```python
from build123d import *

# Parameters (mm, degrees)
SKETCH1_W               = 45
SKETCH1_H               = 24
BOSS_EXTRUDE1_DEPTH     = 5
SKETCH2_W               = 5
SKETCH2_H               = 24
BOSS_EXTRUDE2_DEPTH     = 46
SKETCH3_W               = 45
SKETCH3_H               = 5
BOSS_EXTRUDE3_DEPTH     = 20
CHAMFER2_SIZE           = 45.996850945
CHAMFER2_SIZE_2         = 20
CHAMFER3_SIZE2          = 45.996850945
CHAMFER3_SIZE           = 20
SKETCH4_W               = 5
SKETCH4_H               = 42
BOSS_EXTRUDE4_DEPTH     = 29
CUT_EXTRUDE1_DEPTH      = 75.498322129
CUT_EXTRUDE1_DEPTH_BACK = 75.498322129
SKETCH6_R               = 17
SKETCH7_W               = 46
SKETCH7_H               = 44
CUT_EXTRUDE2_DEPTH      = 75.498322129
SKETCH8_R               = 1.65
CUT_EXTRUDE3_DEPTH      = 75.498322129
SKETCH9_R               = 4.5
CUT_EXTRUDE4_DEPTH      = 75.498322129
FILLET1_R               = 5
SKETCH10_R              = 2.65
CUT_EXTRUDE5_DEPTH      = 10
SKETCH11_R              = 2.65
CUT_EXTRUDE6_DEPTH      = 10
SKETCH12_W              = 45
SKETCH12_H              = 5
BOSS_EXTRUDE5_DEPTH     = 24
SKETCH13_R              = 2.65
CUT_EXTRUDE7_DEPTH      = 10
CUT_EXTRUDE8_DEPTH      = 84.366660003
CUT_EXTRUDE8_DEPTH_BACK = 84.366660003
FILLET2_R               = 2.5


# Some blends are built 0.0001 mm under size
with BuildPart() as part:
    # Sketch1 → Boss-Extrude1 (new body)
    with BuildSketch(Plane.XY):
        with Locations((22.5, 12)):
            Rectangle(SKETCH1_W, SKETCH1_H)
    extrude(amount=BOSS_EXTRUDE1_DEPTH)

    # Sketch2 → Boss-Extrude2 (add)
    with BuildSketch(Plane(origin=(0, 0, 0), x_dir=(-1, 0, 0), z_dir=(0, 0, -1))):
        with Locations((-22.5, 12)):
            Rectangle(SKETCH2_W, SKETCH2_H)
    extrude(amount=BOSS_EXTRUDE2_DEPTH)

    # Sketch3 → Boss-Extrude3 (add)
    with BuildSketch(Plane.XY.offset(5)):
        with Locations((22.5, 2.5)):
            Rectangle(SKETCH3_W, SKETCH3_H)
    extrude(amount=BOSS_EXTRUDE3_DEPTH)

    # Chamfer2
    # the kernel refuses this chamfer: 45.996850945, 20 mm, written as the material it adds along each edge
    with BuildSketch(Plane(origin=(25, 0, 0), x_dir=(-0.015383761930769691, 0, -0.9998816629325978), z_dir=(0, 1, 0))) as chamfer2_piece_1_section:
        Polygon((CHAMFER2_SIZE * 0.999881662927, -CHAMFER2_SIZE * 0.0153837619307), (-CHAMFER2_SIZE_2 * 0.0153837619308, -CHAMFER2_SIZE_2 * 0.999881662933), (0, 0), align=None)
    chamfer2_piece_1 = extrude(amount=24, mode=Mode.PRIVATE)
    chamfer2_piece_1 = split(chamfer2_piece_1, bisect_by=Plane(origin=(45, 12, -15.645189054), z_dir=(-1, 0, 0)), keep=Keep.TOP, mode=Mode.PRIVATE)
    add(chamfer2_piece_1)

    # Chamfer3
    chamfer3_edges = [part.edges().sort_by_distance(p)[0] for p in [
        (20, 12, 0),
    ]]
    chamfer3_side = [part.faces().sort_by_distance(p)[0] for p in [
        (19.6, 12, 0),
    ]]
    chamfer(chamfer3_edges, length=CHAMFER3_SIZE - 0.0001, length2=CHAMFER3_SIZE2 - 0.0001, reference=chamfer3_side[0])  # a hair under: the kernel refuses the full size

    # Sketch4 → Boss-Extrude4 (add)
    with BuildSketch(Plane(origin=(0, 24, 0), x_dir=(1, 0, 0), z_dir=(0, 1, 0))):
        with Locations((22.5, 25)):
            Rectangle(SKETCH4_W, SKETCH4_H)
    extrude(amount=BOSS_EXTRUDE4_DEPTH)

    # Sketch6 → Cut-Extrude1 (cut, two sides: drawn at the far end of the back side and taken through both)
    with BuildSketch(Plane(origin=(25, 0, 0), x_dir=(0, 0, -1), z_dir=(1, 0, 0)).offset(-CUT_EXTRUDE1_DEPTH_BACK)):
        with Locations(Location((25, 32.24, 0), (0, 0, 331.00679558))):
            Circle(SKETCH6_R)
    extrude(amount=CUT_EXTRUDE1_DEPTH + CUT_EXTRUDE1_DEPTH_BACK, mode=Mode.SUBTRACT)

    # Sketch7 → Cut-Extrude2 (cut, through all)
    with BuildSketch(Plane.ZY.offset(-20)):
        with Locations((-23, 31)):
            Rectangle(SKETCH7_W, SKETCH7_H)
    extrude(amount=CUT_EXTRUDE2_DEPTH, mode=Mode.SUBTRACT)

    # Sketch8 → Cut-Extrude3 (cut, through all)
    with BuildSketch(Plane.ZY.offset(-20)):
        with Locations(Location((-40.5, 47.74, 0), (0, 0, 270))):
            Circle(SKETCH8_R)
        with Locations(Location((-9.5, 47.74, 0), (0, 0, 270))):
            Circle(SKETCH8_R)
        with Locations(Location((-9.5, 16.74, 0), (0, 0, 270))):
            Circle(SKETCH8_R)
        with Locations(Location((-40.5, 16.74, 0), (0, 0, 270))):
            Circle(SKETCH8_R)
    extrude(amount=-CUT_EXTRUDE3_DEPTH, mode=Mode.SUBTRACT)

    # Sketch9 → Cut-Extrude4 (cut, through all)
    with BuildSketch(Plane(origin=(25, 0, 0), x_dir=(0, 0, -1), z_dir=(1, 0, 0))):
        with Locations((9.5, 16.74)):
            Circle(SKETCH9_R)
        with Locations((40.5, 16.74)):
            Circle(SKETCH9_R)
    extrude(amount=CUT_EXTRUDE4_DEPTH, mode=Mode.SUBTRACT)

    # Fillet1
    fillet1_edges = [part.edges().sort_by_distance(p)[0] for p in [
        (22.5, 0, -46),
        (22.5, 53, -4),
        (22.5, 53, -46),
    ]]
    fillet(fillet1_edges, radius=FILLET1_R)

    # Sketch10 → Cut-Extrude5 (cut)
    with BuildSketch(Plane.XZ):
        with Locations(Location((22.5, 15, 0), (0, 0, 270))):
            Circle(SKETCH10_R)
    extrude(amount=-CUT_EXTRUDE5_DEPTH, mode=Mode.SUBTRACT)

    # Sketch11 → Cut-Extrude6 (cut)
    with BuildSketch(Plane.XY.offset(5)):
        with Locations((10, 15)):
            Circle(SKETCH11_R)
    extrude(amount=-CUT_EXTRUDE6_DEPTH, mode=Mode.SUBTRACT)

    # Sketch12 → Boss-Extrude5 (add)
    with BuildSketch(Plane(origin=(0, 0, 0), x_dir=(1, 0, 0), z_dir=(0, 1, 0))):
        with Locations((22.5, -27.5)):
            Rectangle(SKETCH12_W, SKETCH12_H)
    extrude(amount=BOSS_EXTRUDE5_DEPTH)

    # Sketch13 → Cut-Extrude7 (cut)
    with BuildSketch(Plane.XY.offset(30)):
        with Locations((22.5, 15)):
            Circle(SKETCH13_R)
    extrude(amount=-CUT_EXTRUDE7_DEPTH, mode=Mode.SUBTRACT)

    # Sketch14 → Cut-Extrude8 (cut, two sides: drawn at the far end of the back side and taken through both)
    with BuildSketch(Plane(origin=(45, 0, 0), x_dir=(0, 0, -1), z_dir=(1, 0, 0)).offset(-CUT_EXTRUDE8_DEPTH_BACK)):
        Polygon((-25, 5), (-26, 5), (-25, 9), align=None)
        Polygon((-5, 5), (-4, 5), (-5, 9), align=None)
    extrude(amount=CUT_EXTRUDE8_DEPTH + CUT_EXTRUDE8_DEPTH_BACK, mode=Mode.SUBTRACT)

    # Fillet2
    # the kernel refuses this fillet: 2.5 mm, written as the material it adds along each edge
    with BuildSketch(Plane(origin=(25, 24, -4), x_dir=(0, 0, 1), z_dir=(-1, 0, 0))) as fillet2_piece_1:
        with BuildLine():
            CenterArc((FILLET2_R, FILLET2_R), FILLET2_R, 180, 90)
            Line((0, FILLET2_R), (0, 0))
            Line((0, 0), (FILLET2_R, 0))
        make_face()
    extrude(amount=5)
    with BuildSketch(Plane(origin=(25, 24, -16.380487567), x_dir=(1, 0, 0), z_dir=(0, 0, 1))) as fillet2_piece_2_section:
        with BuildLine():
            CenterArc((FILLET2_R, FILLET2_R), FILLET2_R, 180, 90)
            Line((0, FILLET2_R), (0, 0))
            Line((0, 0), (FILLET2_R, 0))
        make_face()
    fillet2_piece_2 = extrude(amount=12.380487567, mode=Mode.PRIVATE)
    fillet2_piece_2 = fillet2_piece_2 - Plane(origin=(25.580464588, 32.24, -25), x_dir=(0, -0.48470588235146506, -0.8746772019516044), z_dir=(1, 0, 0)) * Cylinder(17, 35, mode=Mode.PRIVATE)
    add(fillet2_piece_2)
    with BuildSketch(Plane(origin=(25, 24, -52.246850945), x_dir=(0, 1, 0), z_dir=(0, 0, 1))) as fillet2_piece_3_section:
        with BuildLine():
            CenterArc((FILLET2_R, -FILLET2_R), FILLET2_R, 90, 90)
            Line((0, -FILLET2_R), (0, 0))
            Line((0, 0), (FILLET2_R, 0))
        make_face()
    fillet2_piece_3 = extrude(amount=18.627338512, mode=Mode.PRIVATE)
    fillet2_piece_3 = split(fillet2_piece_3, bisect_by=Plane(origin=(25.437853411, 24.621520757, -46), z_dir=(0, 0, 1)), keep=Keep.TOP, mode=Mode.PRIVATE)
    fillet2_piece_3 = split(fillet2_piece_3, bisect_by=Plane(origin=(26.31729653, 24.621520757, -42.967276338), z_dir=(-0.9170600743850381, 0, 0.398749068925444)), keep=Keep.TOP, mode=Mode.PRIVATE)
    fillet2_piece_3 = fillet2_piece_3 - Plane(origin=(25.437853411, 32.24, -25), x_dir=(0, -0.48470588235146506, -0.8746772019516044), z_dir=(1, 0, 0)) * Cylinder(17, 48, mode=Mode.PRIVATE)
    add(fillet2_piece_3)
    with BuildSketch(Plane(origin=(25, 24, -16.380487567), x_dir=(1, 0, 0), z_dir=(0, 0, 1))) as fillet2_piece_4a_section:
        with BuildLine():
            CenterArc((FILLET2_R, FILLET2_R), FILLET2_R, 180, 90)
            Line((0, FILLET2_R), (0, 0))
            Line((0, 0), (FILLET2_R, 0))
        make_face()
    fillet2_piece_4a = extrude(amount=18.630487567, mode=Mode.PRIVATE)
    fillet2_piece_4a = split(fillet2_piece_4a, bisect_by=Plane(origin=(25.565987786, 24.565987786, -4), z_dir=(0, 0, 1)), keep=Keep.TOP, mode=Mode.PRIVATE)
    with BuildSketch(Plane(origin=(31.25, 24, -4), x_dir=(0, 0, 1), z_dir=(-1, 0, 0))) as fillet2_piece_4b_section:
        with BuildLine():
            CenterArc((FILLET2_R, FILLET2_R), FILLET2_R, 180, 90)
            Line((0, FILLET2_R), (0, 0))
            Line((0, 0), (FILLET2_R, 0))
        make_face()
    fillet2_piece_4b = extrude(amount=11.25, mode=Mode.PRIVATE)
    fillet2_piece_4b = split(fillet2_piece_4b, bisect_by=Plane(origin=(25, 24.565987786, -3.434012214), z_dir=(1, 0, 0)), keep=Keep.TOP, mode=Mode.PRIVATE)
    fillet2_piece_4 = fillet2_piece_4a & fillet2_piece_4b
    add(fillet2_piece_4)


solid = part.part
```
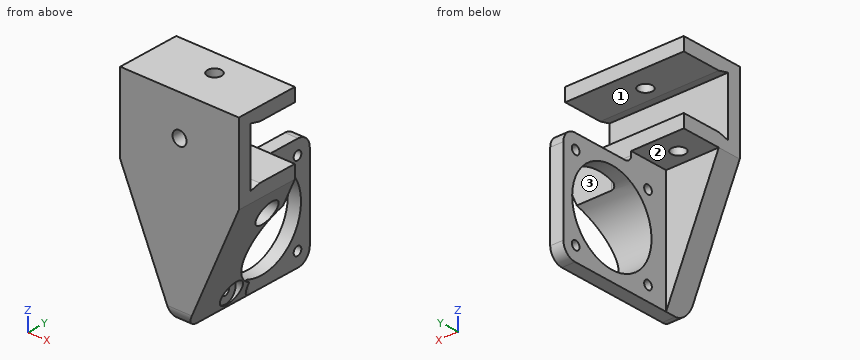
Geometry: final body of the model. Coordinates: model frame, mm. Face numbers are marked on the shaded views. A direction names the side the tool comes from. Give positions to 0.01 mm unless a question says otherwise; leave off trailing zeros. Order: outer loops, then holes, each group sorted by start corner. A loop starts at its lowest first (then second) coordinate and runs counter-clockwise, first axis right, second up. Notation, with made-up numbers: (53.5, 51.5) -> (100.5, 51.5) arc R16 ccw to (100.5, 79.5) -> close; hole circle Ø11 at (8, -2). An arc over 180 degrees is marked (long way). Write each question's results on one line, items separated by ' | '. Start each with the question number.
1) First-contact query: pin 1 (21 mm diameter, centred on y = 31.5, z = -21.5, fed in from +X); pin 2 (3 mm diameter, centred on x = 40, y = 23, fed in from -Z); pin 3 (5.5 mm diameter, centred on x = 22, y = 35.5, fed in from +Z); pin 4 (2.5 mm diameter, centred on x = 21, z = 26.5, fed in from +Y). Flat tips, straight axial feed; report the tip coordinate or a pass-through.
2) Line query: line 1 (Z direction, x = 8, y = 12); line 2 (Y direction, x = 29.25, z = -9.5); line 3 (Z direction, x = 21.15, y = 47.74). Output: solid intervals per line, ascending. Write a range as from..to.
3) Section D-D (x = 11). Return loops of the section in (y, z).
4) Section B-B (y = 32.24). Return loops of the section in (x, z).
5) Section A-A (z = 15). Return loops of the section in (x, y).
6) Set-up query: the marked faces 1, 2 and 3. Return all of +Z, -Z, +X, -X, +Y, -Y with unobstructed straight access to the full face (end or side cutting, diameter ignored); none if empty.
7) Section C-C (x = 21). Count the separate pieces of the cut face and the enclosed holes in it, then the cut area to 3 significant figures.
Calculated:
1) pin 1: through | pin 2: z = -11.82 | pin 3: z = -4 | pin 4: y = 24
2) line 1: 0..5, 25..30 | line 2: 0..12.24, 21.24..24 | line 3: -46..-42.15, -38.85..-31.98, -18.02..-11.15, -7.85..-4
3) outline: (0, -25.3) -> (9, -25.3) -> (9, 0) -> (12.55, 0) -> (12.55, 5) -> (9, 5) -> (5, 4) -> (5, 26) -> (9, 25) -> (24, 25) -> (24, 30) -> (0, 30) -> close; (17.45, 0) -> (24, 0) -> (24, 5) -> (17.45, 5) -> close
4) outline: (20, -46) -> (25, -46) -> (25, -42) -> (20, -42) -> close; (20, -8) -> (25, -8) -> (25, -4) -> (20, -4) -> close
5) outline: (0, 0) -> (19.85, 0) -> (19.85, 5) -> (0, 5) -> close; (25.15, 0) -> (45, 0) -> (45, 5) -> (25.15, 5) -> close
6) face 1: +X, -X, +Y | face 2: -Z, -X, +Y | face 3: +Z, +X, +Y
7) separate pieces: 3 | enclosed holes: 5 | area: 1,660 mm2
